Input: part model. Units: mm. Frame: model coordinates. Face numbers are marked on the shaded views. A direction names the side the tool comes from. Give positions to 0.01 mm unless a question says otherwise; leave off trailing zeros. Write each loop counter-clockwise with the first axis right and the second up, starting at its lowest first coordinate (ties: lowest second). Pieces come first, ordered by that corner, then holes.
```python
from build123d import *

# Parameters (mm, degrees)
F0_W     = 3.175
F0_H     = 2.921
F0_W_2   = 19.05
F0_H_2   = 8.1915
F2_R     = 2.921
F3_DEPTH = 254
F4_SIZE  = 0.254


with BuildPart() as f1:
    # F0 (on Front) → F1 (revolve)
    with BuildSketch(Plane.XZ):
        with Locations((-11.1125, 1.4605)):
            Rectangle(F0_W, F0_H)
        with Locations((0, 1.4605)):
            Rectangle(F0_W_2, F0_H)
        with Locations((11.1125, 1.4605)):
            Rectangle(F0_W, F0_H)
        with Locations((0, 7.01675)):
            Rectangle(F0_W_2, F0_H_2)
    revolve(axis=Axis((0, 0, 0), (1, 0, 0)))

    # F2 (on Front) → F3 (cut, symmetric)
    with BuildSketch(Plane.XZ):
        Circle(F2_R)
    extrude(amount=F3_DEPTH, both=True, mode=Mode.SUBTRACT)

    # F4
    f4_edges = [f1.edges().sort_by_distance(p)[0] for p in [
        (-12.7, 0, -2.921),
        (-9.525, 0, -11.1125),
        (9.525, 0, -11.1125),
        (12.7, 0, -2.921),
    ]]
    chamfer(f4_edges, length=F4_SIZE)


solid = f1.part
```
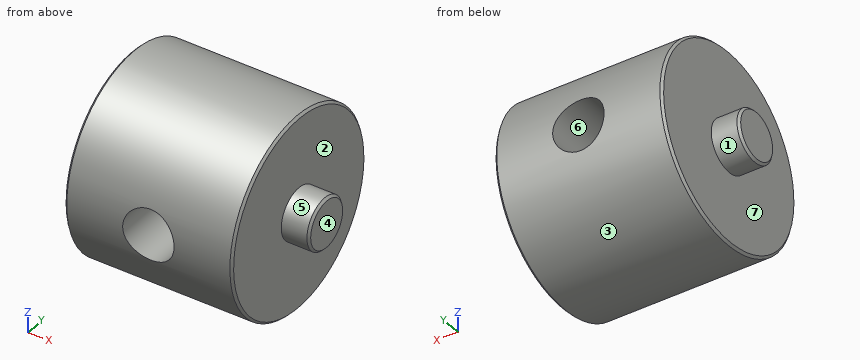
Item 1: Section D-D (x = -5.5). Return loops of the section in (y, z) (1 decimal), and give its area (3 significant figures).
Item 2: Set-up query: the marked faces 1, 2 and 3. Return all of +Z, -Z, +X, -X, +Y, -Y with unobstructed straight access to the full face (end or side cutting, diameter ignored); none if empty.
Item 3: Section C-C (x = 0). Return loops of the section in (y, z) (1 decimal).
Item 4: Pin query (flat end, axial travel): pin 1 (10 mm diameter, centred on y = -7, z = -4.5, fed in from -X) (3 decimals); pin 2 (10 mm diameter, centred on x = 2.5, y = 8, fed in from +Z); pin 3 (3 mm diameter, centred on x = -8.5, y = -4, fed in from +Z). Return the tip coordinate at first contact, or that it passes through.
Item 5: Mould query, pull axis X, two halves, no side actions, for the marked faces 4, 5, 6 and 7. Classes: +X half, -X half, draft (parallel to the pull), parting line (faces both ways), or undercut.
Item 6: Ray query, line 1 (X direction, y = -5, z = 0) (3 decimals); line 2 (X direction, y = 0.5, z = 7.5) (3 decimals); line 3 (Z direction, x = 0, y = -0.5). Return the intervals inside material, ascending.
Solved:
1. outline: circle Ø22.2 at (0, 0)
1. area: 388 mm2
2. face 1: -X
2. face 2: +X
2. face 3: +X, -X
3. outline: (-10.7, -2.9) arc R11.1 ccw to (10.7, -2.9) - close; (-10.7, 2.9) - (10.7, 2.9) arc R11.1 ccw to start
4. pin 1: stops at x = -9.525
4. pin 2: stops at z = 10.7
4. pin 3: stops at z = 10.83
5. face 4: +X half
5. face 5: draft
5. face 6: undercut
5. face 7: -X half
6. line 1: x = -9.525 to -2.921, 2.921 to 9.525
6. line 2: x = -9.525 to 9.525
6. line 3: z = -11.1 to -2.92, 2.92 to 11.1
